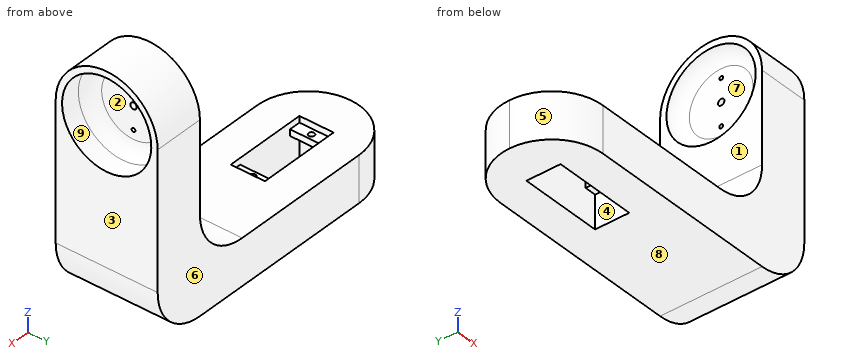
```python
from build123d import *

# Parameters (mm, degrees)
BOSS_EXTRUDE1_DEPTH = 20
SKETCH2_R           = 17.5
CUT_EXTRUDE1_DEPTH  = 12.7
CUT_EXTRUDE2_START  = -4.8
SKETCH3_R           = 17.5
CUT_EXTRUDE2_DEPTH  = 4.8
SKETCH4_R           = 1.25
SKETCH4_R_2         = 0.75
CUT_EXTRUDE3_DEPTH  = 4.8
SKETCH5_W           = 18
SKETCH5_H           = 40
BOSS_EXTRUDE2_DEPTH = 95.4
FILLET1_R           = 20
SKETCH7_W           = 32.5
SKETCH7_H           = 13.4
CUT_EXTRUDE4_DEPTH  = 2.5
FILLET2_R           = 5
FILLET3_R           = 20
SKETCH8_W           = 32.5
SKETCH8_H           = 13.4
CUT_EXTRUDE5_DEPTH  = 13
SKETCH9_R           = 1.15
SKETCH9_W           = 23.6
SKETCH9_H           = 13.4
CUT_EXTRUDE6_DEPTH  = 13


# Some blends are built 0.0001 mm under size
with BuildPart() as part:
    # Sketch1 → Boss-Extrude1 (new body)
    with BuildSketch(Plane(origin=(0, 0, 0), x_dir=(0, 0, -1), z_dir=(1, 0, 0))):
        with BuildLine():
            Line((73.32, 20), (0, 20))
            ThreePointArc((0, 20), (14.142135624, 14.142135624), (20, 0))
            ThreePointArc((20, 0), (14.142135624, -14.142135624), (0, -20))
            Line((0, -20), (73.32, -20))
            Line((73.32, -20), (73.32, 20))
        make_face()
        with BuildLine():
            ThreePointArc((20, 0), (14.142135624, 14.142135624), (0, 20))
            Line((0, 20), (0, -20))
            ThreePointArc((0, -20), (14.142135624, -14.142135624), (20, 0))
        make_face()
        with BuildLine():
            Line((0, -20), (0, 20))
            ThreePointArc((0, 20), (-20, 0), (0, -20))
        make_face()
    extrude(amount=BOSS_EXTRUDE1_DEPTH)

    # Sketch2 → Cut-Extrude1 (cut)
    with BuildSketch(Plane(origin=(20, 0, 0), x_dir=(0, 0, -1), z_dir=(1, 0, 0))):
        Circle(SKETCH2_R)
    extrude(amount=-CUT_EXTRUDE1_DEPTH, mode=Mode.SUBTRACT)

    # Sketch3 → Cut-Extrude2 (cut)
    with BuildSketch(Plane.ZY.offset(CUT_EXTRUDE2_START)):
        with Locations(Location((0, 0, 0), (0, 0, 180))):
            Circle(SKETCH3_R)
    extrude(amount=CUT_EXTRUDE2_DEPTH, mode=Mode.SUBTRACT)

    # Sketch4 → Cut-Extrude3 (cut)
    with BuildSketch(Plane.ZY.offset(-4.8)):
        Circle(SKETCH4_R)
        with Locations((-9, 0)):
            Circle(SKETCH4_R_2)
        with Locations((9, 0)):
            Circle(SKETCH4_R_2)
    extrude(amount=-CUT_EXTRUDE3_DEPTH, mode=Mode.SUBTRACT)

    # Sketch5 → Boss-Extrude2 (add)
    with BuildSketch(Plane.ZY):
        with Locations((-64.32, 0)):
            Rectangle(SKETCH5_W, SKETCH5_H)
    extrude(amount=BOSS_EXTRUDE2_DEPTH)

    # Fillet1
    fillet1_edges = [part.edges().sort_by_distance(p)[0] for p in [
        (-95.4, -20, -64.32),
        (-95.4, 20, -64.32),
    ]]
    fillet(fillet1_edges, radius=FILLET1_R - 0.0001)  # a hair under: the kernel refuses the full size

    # Sketch7 → Cut-Extrude4 (cut)
    with BuildSketch(Plane.XY.offset(-55.32)):
        with Locations((-63.1, 0)):
            Rectangle(SKETCH7_W, SKETCH7_H)
    extrude(amount=-CUT_EXTRUDE4_DEPTH, mode=Mode.SUBTRACT)

    # Fillet2
    # the kernel refuses this fillet: 5 mm, written as the material it adds along each edge
    with BuildSketch(Plane(origin=(7.3, 0, 0), x_dir=(0, 0, -1), z_dir=(0, -1, 0))) as fillet2_piece_1:
        with BuildLine():
            CenterArc((17.5 - FILLET2_R, FILLET2_R), FILLET2_R, 270, 90)
            Line((17.5 - FILLET2_R, 0), (17.5 - FILLET2_R, -FILLET2_R * 0.02))
            Line((17.5 - FILLET2_R, -FILLET2_R * 0.02), (17.5 + FILLET2_R * 0.02, -FILLET2_R * 0.02))
            Line((17.5 + FILLET2_R * 0.02, -FILLET2_R * 0.02), (17.5 + FILLET2_R * 0.02, FILLET2_R))
            Line((17.5 + FILLET2_R * 0.02, FILLET2_R), (17.5, FILLET2_R))
        make_face()
    revolve(axis=Axis((7.3, 0, 0), (1, 0, 0)))
    with BuildSketch(Plane(origin=(4.8, 0, 0), x_dir=(0, 0, -1), z_dir=(0, 1, 0))) as fillet2_piece_2:
        with BuildLine():
            CenterArc((12.504001601, 5), FILLET2_R, 270, 87.707557224)
            Line((12.504001601, 0), (12.504001601, -0.1))
            Line((12.504001601, -0.1), (17.5, -0.1))
            Line((17.5, -0.1), (17.6, 0))
            ThreePointArc((17.6, 0), (17.6, 2.4), (17.599919968, 4.796))
            Line((17.599919968, 4.796), (17.5, 4.8))
        make_face()
    revolve(axis=Axis((4.8, 0, 0), (-1, 0, 0)))

    # Fillet3
    fillet3_edges = [part.edges().sort_by_distance(p)[0] for p in [
        (20, 0, -73.32),
        (0, 0, -55.32),
    ]]
    fillet(fillet3_edges, radius=FILLET3_R)

    # Sketch8 → Cut-Extrude5 (cut)
    with BuildSketch(Plane(origin=(0, 0, -73.32), x_dir=(-1, 0, 0), z_dir=(0, 0, -1))):
        with Locations((63.1, 0)):
            Rectangle(SKETCH8_W, SKETCH8_H)
    extrude(amount=-CUT_EXTRUDE5_DEPTH, mode=Mode.SUBTRACT)

    # Sketch9 → Cut-Extrude6 (cut)
    with BuildSketch(Plane.XY.offset(-57.82)):
        with Locations((-77, 0)):
            Circle(SKETCH9_R)
        with Locations((-49.2, 0)):
            Circle(SKETCH9_R)
        with Locations((-63.1, 0)):
            Rectangle(SKETCH9_W, SKETCH9_H)
    extrude(amount=-CUT_EXTRUDE6_DEPTH, mode=Mode.SUBTRACT)


solid = part.part
```
Input: part model. Units: mm. Frame: model coordinates. Face numbers are marked on the shaded views. A direction names the side the tool comes from. Round coordinates to 2 decimals unless told otherwise and drop trailing zeros. Loops run counter-clockwise (first coordinate to the right, second up) from the corner with the lowest first, then second, coordinate; pieces in that order, holes last.
1) Pin query (flat end, axial travel): pin 1 (1.3 mm diameter, centred on x = -48, y = 2.5, fed in from -Z); pin 2 (1.5 mm diameter, centred on x = -69, y = 6, fed in from +Z); pin 3 (1.4 mm diameter, centred on x = -49.2, y = 0, fed in from +Z); pin 4 (2.5 mm diameter, centred on y = -2, z = -59, fed in from +X). Return the tip coordinate at first contact, or that it passes through.
Ans:
pin 1: stops at z = -60.32
pin 2: stops at z = -55.32
pin 3: passes through
pin 4: stops at x = 19.5
2) Material intervals for line 1 (Z direction, x = -55.5, y = 17); line 2 (Y direction, x = -49.2, z = -58.55); line 3 (X direction, y = 3.5, z = -35), sorted ascending.
Ans:
line 1: z = -73.32 to -55.32
line 2: y = -20 to -1.15, 1.15 to 20
line 3: x = 0 to 20
3) Set-up query: the marked faces 1, 2, 3, 4 and 5. Return all of +Z, -Z, +X, -X, +Y, -Y with unobstructed straight access to the full face (end or side cutting, diameter ignored); none if empty.
Ans:
face 1: +Z, -X, +Y, -Y
face 2: +X
face 3: +Z, -Z, +X, +Y, -Y
face 4: -Z
face 5: +Z, -Z, -X, -Y
4) Section query C-C on z = -52. Return the cut outline in (x, y), plus the area to 3 significant figures.
Ans:
outline: (-8.96, -20) - (20, -20) - (20, 20) - (-8.96, 20) - close
area: 1,160 mm2
5) Pull-direction query (Z, two-part tool) for the marked faces 6, 7, 8 and 9; classes: released by +Z, released by -Z, zero draft, split by the parting line, or undercut.
Ans:
face 6: zero draft
face 7: undercut
face 8: released by -Z
face 9: undercut
6) Section query B-B on x = -34.5. Return the cut outline in (y, z), plus the area to 3 significant figures.
Ans:
outline: (-20, -73.32) - (20, -73.32) - (20, -55.32) - (-20, -55.32) - close
area: 720 mm2
7) Section query A-A on x = -67. Return the cut outline in (y, z).
Ans:
outline: (-20, -73.32) - (-6.7, -73.32) - (-6.7, -55.32) - (-20, -55.32) - close; (6.7, -73.32) - (20, -73.32) - (20, -55.32) - (6.7, -55.32) - close
